Autodesk Inventor part; units mm, degrees
ref_plane "YZ Plane" through (0, 0, 0) normal (1, 0, 0) x (0, 1, 0)
ref_plane "XZ Plane" through (0, 0, 0) normal (0, 1, 0) x (-1, 0, 0)
ref_plane "XY Plane" through (0, 0, 0) normal (0, 0, 1) x (1, 0, 0)
sketch "Sketch1" plane through (0, 0, 0) normal (0, 0, 1) x (1, 0, 0)
  circle A0 centre (0, 0) radius 1.5
  circle A1 centre (0, 0) radius 2.7
  dimension "d0" = 3
  dimension "d5" = 5.4
extrude "Extrusion1" add sketch "Sketch1" along normal blind 20.5 contours A0
extrude "Extrusion2" add sketch "Sketch1" against normal blind 3 contours A0 | A1
thread "Thread2"
fillet "Fillet1" radius 0.25 1 edges at (-2.7, 0, -3)
sketch "Sketch2" plane through (0, 0, -3) normal (0, 0, -1) x (-1, 0, 0)
  circle A0 centre (0, 0) radius 1.5
  line L0 (-1.5, 0) -> (-0.75, 1.299)
  line L1 (-0.75, 1.299) -> (0.75, 1.299)
  line L2 (0.75, 1.299) -> (1.5, 0)
  line L3 (1.5, 0) -> (0.75, -1.299)
  line L4 (0.75, -1.299) -> (-0.75, -1.299)
  line L5 (-0.75, -1.299) -> (-1.5, 0)
extrude "Extrusion3" cut sketch "Sketch2" against normal blind 2 contours L3 L4 L5 L0 L1 L2
properties part number "COTS_GENERIC_Solenoid_Actuator_Push_Rod_M3"
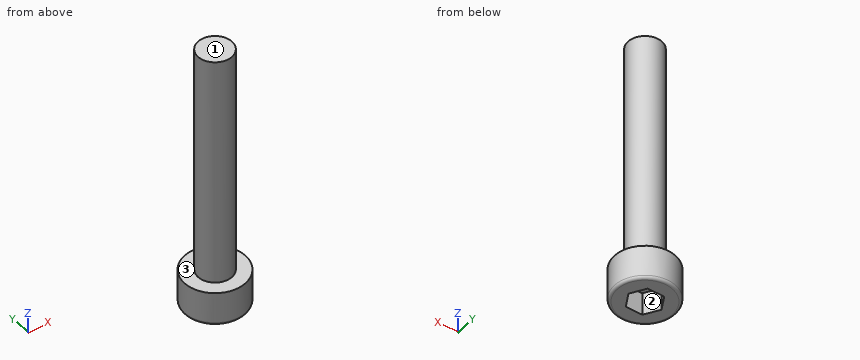
Read the model definition and answer for the solid it produces. Units are mm, in the model's axes. Face numbers are marked on the shaded views. A direction names the side the tool comes from. Give positions to 0.01 mm unless a question says otherwise; leave off trailing zeros. Write each loop counter-clockwise with the first axis right and the second up, starting at its lowest first coordinate (ties: lowest second). Pieces come first, ordered by that corner, then holes. Notation, with made-up numbers: M -28.5,63 L 1.5,63 A4 cw 1.5,70 Z; hole C 81,71 d7. An arc over 180 degrees is marked long. One line per item, written item: value. Start each with the question number.
(1) Flat-ended cylindrical pins translate along their axes: pin 1 Ø1 at (x, z) = (-1.5, 8) entering from +Y; pin 2 Ø3 at (y, z) = (2, 3.5) entering from +X. Find the tip coordinate at first contact, or state that the pin passes through.
(2) Find section A-A (x = 0). Determine the outline of the cut face in (y, z), plus the area to 3 significant figures.
(3) A tool of negligible diameter and unlimited length cuts with its end or side. For the marked faces 1, 2 and 3, from which of +Z, -Z, +X, -X, +Y, -Y can it reach the whole face along a straight path? Write none if from no direction.
(4) Find the intervals of material crossed by line 1 (Z direction, x = -0.45, y = 0.5); line 2 (Z direction, x = -1.2, y = -2.05); line 3 (X direction, y = -1.3, z = 5.75), in increasing order.
(5) Find section B-B (z = 0.5). Determine the outline of the cut face in (x, y).
Results below:
1. pin 1: stops at y = 1.12
1. pin 2: stops at x = 1.41
2. outline: M -2.7,-2.75 A0.25 ccw -2.45,-3 L -1.3,-3 L -1.3,-1 L 1.3,-1 L 1.3,-3 L 2.45,-3 A0.25 ccw 2.7,-2.75 L 2.7,0 L 1.5,0 L 1.5,20.5 L -1.5,20.5 L -1.5,0 L -2.7,0 Z
2. area: 72.5 mm^2
3. face 1: +Z, +X, -X, +Y, -Y
3. face 2: -Z
3. face 3: +Z
4. line 1: z = -1 to 20.5
4. line 2: z = -3 to 0
4. line 3: x = -0.75 to 0.75
5. outline: C 0,0 d3
